Design review of the part built by this model. Coordinates are the model's own, in mm. Face numbers are marked on the shaded views. A direction names the side the tool comes from. Coordinates: 2 decimals unless noted, no trailing zeros. Order: outer loops, then holes, each group sorted by start corner. A loop starts at its lowest first (then second) coordinate and runs counter-clockwise, first axis right, second up. Notation, with made-up numbers: M -6.75,7.5 L 45.25,7.5 A19 ccw 45.25,40.5 Z; hole C 69,-17 d1. An arc over 180 degrees is marked long. Answer as a JSON object with one key per item and string values.
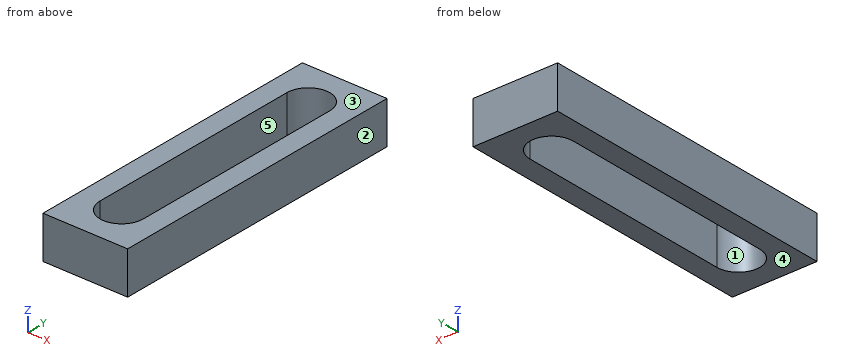
from build123d import *

# Parameters (mm, degrees)
SKETCH1_W               = 50.8
SKETCH1_H               = 182.629999942
BOSS_EXTRUDE1_DEPTH     = 25.4
CUT_EXTRUDE1_DEPTH      = 108.537106246
CUT_EXTRUDE1_DEPTH_BACK = 108.537106246


with BuildPart() as part:
    # Sketch1 → Boss-Extrude1 (new body)
    with BuildSketch(Plane.XY):
        with Locations((25.4, 0)):
            Rectangle(SKETCH1_W, SKETCH1_H)
    extrude(amount=BOSS_EXTRUDE1_DEPTH)

    # Sketch2 → Cut-Extrude1 (cut, two sides: drawn at the far end of the back side and taken through both)
    with BuildSketch(Plane.XY.offset(25.4).offset(-CUT_EXTRUDE1_DEPTH_BACK)):
        with BuildLine():
            Line((38.3, 65.714999971), (38.3, -65.714999971))
            ThreePointArc((38.3, -65.714999971), (25.4, -78.614999971), (12.5, -65.714999971))
            Line((12.5, -65.714999971), (12.5, 65.714999971))
            ThreePointArc((12.5, 65.714999971), (25.4, 78.614999971), (38.3, 65.714999971))
        make_face()
    extrude(amount=CUT_EXTRUDE1_DEPTH + CUT_EXTRUDE1_DEPTH_BACK, mode=Mode.SUBTRACT)


solid = part.part
1) Add section C-C (z = 20.25). State the section outline as (x, y) points (3 decimals).
Taken from the geometry:
{"outline": "M 0,-91.315 L 50.8,-91.315 L 50.8,91.315 L 0,91.315 Z; hole M 12.5,-65.715 A12.9 ccw 38.3,-65.715 L 38.3,65.715 A12.9 ccw 12.5,65.715 Z"}
2) Add section B-B (x = 25.4). State the section outline as (y, z) points (3 decimals).
Taken from the geometry:
{"outline": "M -91.315,0 L -78.615,0 L -78.615,25.4 L -91.315,25.4 Z; M 78.615,0 L 91.315,0 L 91.315,25.4 L 78.615,25.4 Z"}
3) Tool access review of the marked faces 4 and 5: name each direction out of +Z, -Z, +X, -X, +Y, -Y from which nothing blocks a thin tool from reaching the whole face with its end or side.
Taken from the geometry:
{"face 4": "-Z, +X, -X, +Y, -Y", "face 5": "+Z, -Z"}
4) To check wall thickness, follow L1, parallel to X at y = 36.5, z = 8.25; L2, parallel to Y at x = 31, z = 10.25 (3 decimals); L3, parallel to Y at x = 31.5, z = 18 (3 decimals). State the ranges of each line that lie inside material, in increasing order.
Taken from the geometry:
{"L1": "x = 0 to 12.5, 38.3 to 50.8", "L2": "y = -91.315 to -77.336, 77.336 to 91.315", "L3": "y = -91.315 to -77.082, 77.082 to 91.315"}
5) Mouldability with a two-part tool opening along X and no side actions: class the marked faces 1, 2 and 3 as released by +X, released by -X, zero draft, split by the parting line, or undercut.
Taken from the geometry:
{"face 1": "undercut", "face 2": "released by +X", "face 3": "zero draft"}
6) Add section A-A (y = 0). State the section outline as (x, z) points.
Taken from the geometry:
{"outline": "M 0,0 L 12.5,0 L 12.5,25.4 L 0,25.4 Z; M 38.3,0 L 50.8,0 L 50.8,25.4 L 38.3,25.4 Z"}
